Work out the finished part from the listing and answer in its coordinate system (mm). Coordinates: 2 decimals unless noted, no trailing zeros. Order: outer loops, then holes, each group sorted by start corner. A loop starts at its lowest first (then second) coordinate and runs counter-clockwise, first axis right, second up. Notation, with made-up numbers: (-20, -32.5) -> (17, -32.5) arc R37 ccw to (17, 4.5) -> close; hole circle Ø11 at (-30, 75.25). An arc over 180 degrees is marked (long way). Write item = value, one per line. Start each with the question number.
Q1. Flat-ended cylindrical pins translate along their axes: pin 1 (2 mm diameter, centred on x = -0.5, z = -16.5, fed in from -Y); pin 2 (10 mm diameter, centred on y = 15, z = -20, fed in from +X); pin 3 (2 mm diameter, centred on y = 29, z = -20.5, fed in from -X); pin 4 (3 mm diameter, centred on x = -1.5, z = -19, fed in from +Y). Find the tip coordinate at first contact, or state that the pin passes through.
Q2. The part is cut by section C-C, the plane z = -35. Determine the outline of the cut face in (x, y).
Q3. The part is cut by section A-A, the plane x = -5. Determine the outline of the cut face in (y, z), plus the area to 3 significant figures.
Q4. Straight lines are drawn through the part: L1, parallel to X at y = 27.5, z = -40.5; L2, parallel to Z at x = -0.25, y = 29.5; L3, parallel to Y at x = -6.5, z = -4. For each, find the intervals that lie inside material, in ascending order. Write a range as from..to.
Q5. The part is cut by section B-B, the plane y = 0. Determine the outline of the cut face in (x, z).
Q6. The part is cut by section D-D, the plane y = 16. Determine the outline of the cut face in (x, z), plus the area to 3 significant figures.
Autodesk Inventor part; units mm, degrees
ref_plane "YZ Plane" through (0, 0, 0) normal (1, 0, 0) x (0, 1, 0)
ref_plane "XZ Plane" through (0, 0, 0) normal (0, 1, 0) x (-1, 0, 0)
ref_plane "XY Plane" through (0, 0, 0) normal (0, 0, 1) x (1, 0, 0)
sketch "Sketch1" plane through (0, 0, 0) normal (0, 0, 1) x (1, 0, 0)
  circle A0 centre (0, 0) radius 6.35
  dimension "d0" = 12.7
extrude "Extrusion1" add sketch "Sketch1" against normal blind 50.8
sketch "Sketch2" plane through (0, 0, 0) normal (0, 0, 1) x (1, 0, 0)
  circle A0 centre (0, 0) radius 7.4295
  dimension "d3" = 14.859
extrude "Extrusion3" add sketch "Sketch2" against normal blind 6.35
sketch "Sketch3" plane through (0, 0, 0) normal (1, 0, 0) x (0, 1, 0)
  line L0 (-6.35, -50.8) -> (6.35, -50.8)
  line L1 (0, -50.8) -> (50.8, -50.8)
  line L2 (50.8, -50.8) -> (50.8, -19.05)
  line L3 (50.8, -19.05) -> (0, -19.05)
  line L4 (0, -19.05) -> (0, -50.8)
  line L5 (7.4295, 0) -> (-7.4295, 0)
  point P0 (0, 0)
  dimension "d8" = 19.05
  dimension "d9" = 50.8
extrude "Extrusion4" add sketch "Sketch3" along normal mid plane 0.635
properties part number "portionOfShade" material "PC/ABS Plastic"
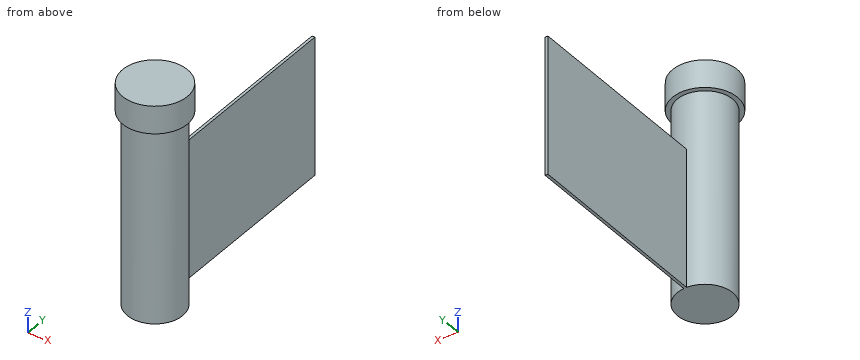
Model answer:
q1.pin_1 = -6.35
q1.pin_2 = 0.32
q1.pin_3 = -0.32
q1.pin_4 = 50.8
q2.outline = (-0.32, 6.34) arc R6.35 ccw (long way) to (0.32, 6.34) -> (0.32, 50.8) -> (-0.32, 50.8) -> close
q3.outline = (-5.5, -6.35) -> (-3.91, -6.35) -> (-3.91, -50.8) -> (3.91, -50.8) -> (3.91, -6.35) -> (5.5, -6.35) -> (5.5, 0) -> (-5.5, 0) -> close
q3.area = 418 mm2
q4.L1 = -0.32..0.32
q4.L2 = -50.8..-19.05
q4.L3 = -3.6..3.6
q5.outline = (-7.43, -6.35) -> (-6.35, -6.35) -> (-6.35, -50.8) -> (6.35, -50.8) -> (6.35, -6.35) -> (7.43, -6.35) -> (7.43, 0) -> (-7.43, 0) -> close
q6.outline = (-0.32, -50.8) -> (0.32, -50.8) -> (0.32, -19.05) -> (-0.32, -19.05) -> close
q6.area = 20.2 mm2
